Design review of the part shown in the three views and the two pictorial views. Dimensions are in mm from the part's minimum x, y and z. Coordinates: 2 decimals unless noted, no trailing zeros. Loops run counter-clockwise (first coordinate to the right, second up) from the corner with the lowest first, then second, coordinate; pieces in that order, holes last. Notation, with made-up numbers: (73, -13.5) -> (122, -13.5) arc R19 cw to (122, 1.5) -> close; hole circle Ø6 at (11.25, 66.5). An arc over 180 degrees is marked (long way). Use CSV: the item, a comma, the result in double quotes.
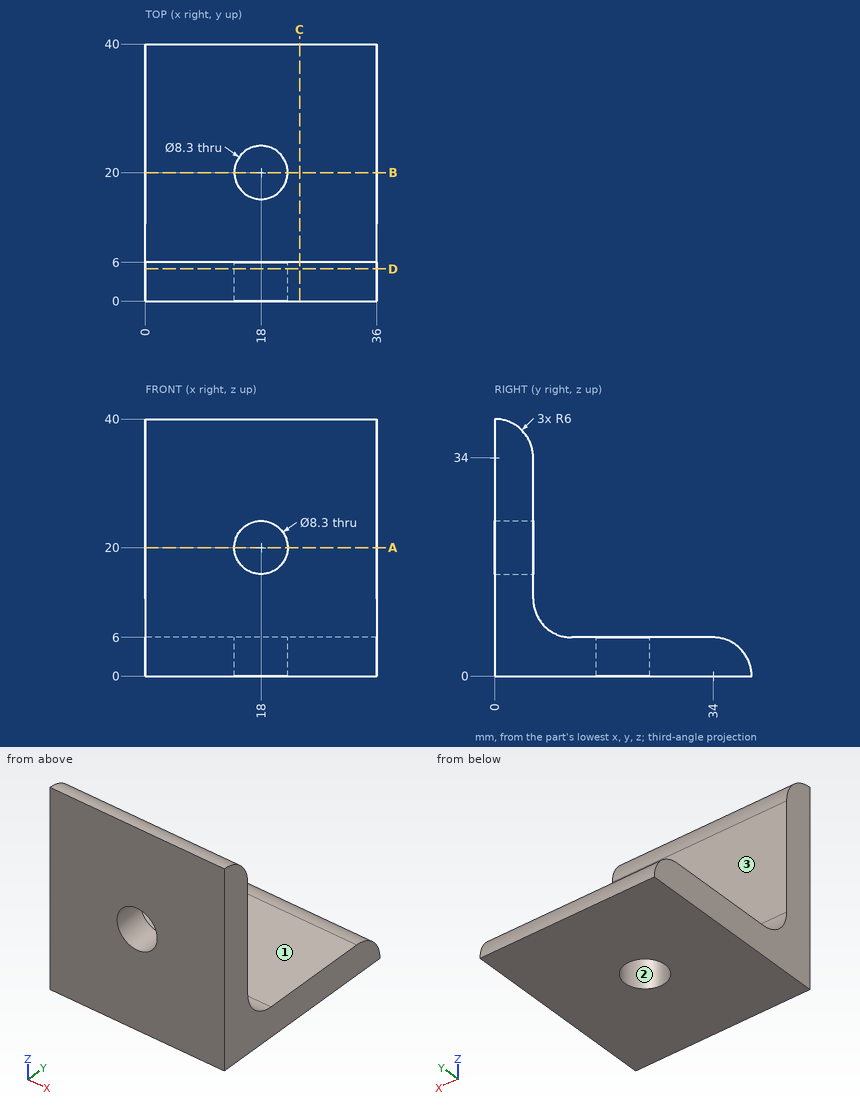
Item 1: Add section C-C (x = 24). Give the boundary of the cut face in (y, z), then the cut area to 3 significant figures.
Checked values:
outline,"(0, 0) -> (40, 0) arc R6 ccw to (34, 6) -> (12, 6) arc R6 cw to (6, 12) -> (6, 34) arc R6 ccw to (0, 40) -> close"
area,"436 mm^2"
Item 2: Clearance check with flat-ended pins moving along their axes: pin 1 (6.5 mm diameter, centred on x = 17, y = 19, fed in from +Z); pin 2 (6 mm diameter, centred on x = 15.5, z = 20.5, fed in from +Y). State where each tip first meets the part, or that it passes through.
Checked values:
pin 1,"z = 6"
pin 2,"y = 6"
Item 3: To check wall thickness, follow line 1 along X through (y, z) = (20, 2); line 2 along Z through (x, y) = (27.5, 30.5). State the ranges of each line that lie inside material, in increasing order.
Checked values:
line 1,"0 to 13.85, 22.15 to 36"
line 2,"0 to 6"
Item 4: Draft analysis for pull direction Y (two halves, no side actions). For the marked faces 1, 2 and 3, state which applies: pulls with the +Y half, pulls with the -Y half, needs draft (parallel to the pull), parting line crosses it, or undercut.
Checked values:
face 1,"needs draft"
face 2,"undercut"
face 3,"pulls with the +Y half"
Item 5: Add section D-D (y = 5). Give the boundary of the cut face in (x, z), then the cut area to 3 significant figures.
Checked values:
outline,"(0, 0) -> (36, 0) -> (36, 37.32) -> (0, 37.32) -> close; hole circle Ø8.3 at (18, 20)"
area,"1,290 mm^2"
Item 6: Add section A-A (z = 20). Give the boundary of the cut face in (x, y), then the cut area to 3 significant figures.
Checked values:
outline,"(0, 0) -> (13.85, 0) -> (13.85, 6) -> (0, 6) -> close; (22.15, 0) -> (36, 0) -> (36, 6) -> (22.15, 6) -> close"
area,"166 mm^2"
